from build123d import *

# Parameters (mm, degrees)
SKETCH1_W           = 19.05
SKETCH1_H           = 50
SKETCH1_R           = 2.1
BOSS_EXTRUDE1_DEPTH = 3.175
SKETCH2_W           = 4.445
SKETCH2_H           = 50
BOSS_EXTRUDE2_DEPTH = 3.175
CUT_EXTRUDE1_DEPTH  = 3.175
FILLET1_R           = 3.175


with BuildPart() as part:
    # Sketch1 → Boss-Extrude1 (new body)
    with BuildSketch(Plane.XY):
        with Locations((-15.475, 0)):
            Rectangle(SKETCH1_W, SKETCH1_H)
        with Locations((-10, 0)):
            Circle(SKETCH1_R, mode=Mode.SUBTRACT)
    extrude(amount=BOSS_EXTRUDE1_DEPTH)

    # Sketch2 → Boss-Extrude2 (add)
    with BuildSketch(Plane.XY.offset(3.175)):
        with Locations((-27.2225, 0)):
            Rectangle(SKETCH2_W, SKETCH2_H)
    extrude(amount=-BOSS_EXTRUDE2_DEPTH)

    # Sketch3 → Cut-Extrude1 (cut)
    with BuildSketch(Plane.XY.offset(3.175)):
        with BuildLine():
            Line((-25.9525, -15.475), (-25.9525, -21.825))
            ThreePointArc((-25.9525, -21.825), (-26.905, -22.7775), (-27.8575, -21.825))
            Line((-27.8575, -21.825), (-27.8575, -15.475))
            ThreePointArc((-27.8575, -15.475), (-26.905, -14.5225), (-25.9525, -15.475))
        make_face()
        with BuildLine():
            Line((-25.9525, 15.475), (-25.9525, 21.825))
            ThreePointArc((-25.9525, 21.825), (-26.905, 22.7775), (-27.8575, 21.825))
            Line((-27.8575, 21.825), (-27.8575, 15.475))
            ThreePointArc((-27.8575, 15.475), (-26.905, 14.5225), (-25.9525, 15.475))
        make_face()
    extrude(amount=-CUT_EXTRUDE1_DEPTH, mode=Mode.SUBTRACT)

    # Fillet1
    fillet1_edges = [part.edges().sort_by_distance(p)[0] for p in [
        (-29.445, -25, 1.5875),
        (-29.445, 25, 1.5875),
        (-5.95, 25, 1.5875),
        (-5.95, -25, 1.5875),
    ]]
    fillet(fillet1_edges, radius=FILLET1_R)


solid = part.part
Verification items for the finished model (mm, model axes). A direction names the side the tool comes from. Coordinates: 2 decimals unless noted, no trailing zeros. Order: outer loops, then holes, each group sorted by start corner. A loop starts at its lowest first (then second) coordinate and runs counter-clockwise, first axis right, second up. Notation, with made-up numbers: (30.5, -8.5) -> (53.5, -8.5) arc R9 cw to (53.5, -3.5) -> close; hole circle Ø4 at (87.25, 55.25). An arc over 180 degrees is marked (long way). Put each result on its own line as item: value. Start each with the question number.
1. Material ranges on L1, parallel to Y at x = -10, z = 2.55; L2, parallel to Y at x = -11.25, z = 2.7, recorded low to high. Write a range as [from, to].
2. Mould release check, pull along Y, two halves, no side actions. Record for faces 3 (the flat face through (-5.95, 0, 2)), 4 (the cylindrical face through (-26.884, 22.777, 1.61)), 5 (the flat face through (-18, 25, 2)): released by +Y, released by -Y, zero draft, split by the parting line, or undercut.
3. Access from +Z, -Z, +X, -X, +Y, -Y to the whole of each face (thin tool, end or side, straight path). Record for faces 1 (the cylindrical face through (-26.926, 14.523, 1.61)), 2 (the flat face through (-18, 0, 3.175)).
4. Cross-section at A-A, the plane y = 0. Record the boundary of the cut face in (x, z) (3 decimals), then the cut area to 3 significant figures.
5. Cross-section at B-B, the plane x = -10. Record the boundary of the cut face in (y, z) (3 decimals).
6. Cross-section at C-C, the plane z = 2.1. Count the separate pieces of the cut face and the enclosed holes in it, then the cut area to 3 significant figures.
Computed:
1. L1: [-25, -2.1], [2.1, 25]
1. L2: [-25, -1.69], [1.69, 25]
2. face 3: zero draft
2. face 4: undercut
2. face 5: released by +Y
3. face 1: +Z, -Z
3. face 2: +Z, +X, -X, +Y, -Y
4. outline: (-29.445, 0) -> (-12.1, 0) -> (-12.1, 3.175) -> (-29.445, 3.175) -> close; (-7.9, 0) -> (-5.95, 0) -> (-5.95, 3.175) -> (-7.9, 3.175) -> close
4. area: 61.3 mm2
5. outline: (-25, 0) -> (-2.1, 0) -> (-2.1, 3.175) -> (-25, 3.175) -> close; (2.1, 0) -> (25, 0) -> (25, 3.175) -> (2.1, 3.175) -> close
6. separate pieces: 1
6. enclosed holes: 3
6. area: 1,120 mm2
